```python
from build123d import *

# Parameters (mm, degrees)
F1_DEPTH = 9.8
F2_W     = 22.898962
F2_H     = 1.623713
F3_DEPTH = 18


with BuildPart() as f1:
    # F0 (on Top) → F1 (new body)
    with BuildSketch(Plane.XY):
        Polygon((30.061033, 31.619072), (-30.061033, 31.619072), (-16.680207, -13.655773), (-13.930722, -13.655773), (0, -13.655773), (13.930722, -13.655773), (16.680207, -13.655773), align=None)
        Polygon((-17.066102, 6.705488), (-22.912372, 26.4867), (22.912372, 26.4867), (17.066102, 6.705488), (0, 6.705488), align=None, mode=Mode.SUBTRACT)
        Polygon((0, -13.655773), (-13.930722, -13.655773), (-13.930722, -74.694335), (0, -74.694335), (13.930722, -74.694335), (13.930722, -13.655773), align=None)
    extrude(amount=F1_DEPTH)

    # F2 (on face) → F3 (cut)
    with BuildSketch(Plane(origin=(0, 6.705488, 0), x_dir=(-1, 0, 0), z_dir=(0, 1, 0))):
        with Locations((-0.274213, 4.465245)):
            Rectangle(F2_W, F2_H)
    extrude(amount=-F3_DEPTH, mode=Mode.SUBTRACT)


solid = f1.part
```
The model under review builds one solid part; all positions refer to its coordinate system, in mm. A direction names the side the tool comes from. Round coordinates to 2 decimals unless told otherwise and drop trailing zeros. Write each loop counter-clockwise with the first axis right and the second up, starting at its lowest first coordinate (ties: lowest second). Pieces come first, ordered by that corner, then holes. Notation, with made-up numbers: (-15.5, 9.25) - (-4.5, 9.25) arc R23 ccw to (-4.5, 45.25) - close; hole circle Ø11 at (78.25, -34.75). An arc over 180 degrees is marked (long way). One line per question, with ' | ' between items.
Item 1: Add section A-A, the plane x = 3.5. Give the boundary of the cut face in (y, z), then the cut area to 3 significant figures.
Resolved:
outline: (-74.69, 0) - (6.71, 0) - (6.71, 3.65) - (-11.29, 3.65) - (-11.29, 5.28) - (6.71, 5.28) - (6.71, 9.8) - (-74.69, 9.8) - close; (26.49, 0) - (31.62, 0) - (31.62, 9.8) - (26.49, 9.8) - close | area: 819 mm2
Item 2: Add section B-B, the plane y = 22. Give the boundary of the cut face in (x, z), then the cut area to 3 significant figures.
Resolved:
outline: (-27.22, 0) - (-21.59, 0) - (-21.59, 9.8) - (-27.22, 9.8) - close; (21.59, 0) - (27.22, 0) - (27.22, 9.8) - (21.59, 9.8) - close | area: 110 mm2
Item 3: For faces 1 (the face through (0, 26.487, 5)), 2 (the face through (13.931, -45, 5)), 3 (the face through (0, -74.694, 5)), 4 (the face through (0, -2, 5.277)), 5 (the face through (-13.931, -44, 5)), list the 3-axis set-ups (+Z, -Z, +X, -X, +Y, -Y) from which the entire face can be reached by the end or side of a thin tool; tool diameter is ignored.
Resolved:
face 1: +Z, -Z | face 2: +Z, -Z, +X, -Y | face 3: +Z, -Z, +X, -X, -Y | face 4: none | face 5: +Z, -Z, -X, -Y
Item 4: The part is to be moulded in two halves that separate along Y. For faces 6 (the face through (20.03, 16.73, 4.83)), 7 (the face through (-15, -13.656, 5)), 8 (the face through (0, -21, 9.8)), say which applies: pulls with the +Y half, pulls with the -Y half, needs draft (parallel to the pull), parting line crosses it, or undercut.
Resolved:
face 6: undercut | face 7: pulls with the -Y half | face 8: needs draft
Item 5: To check wall thickness, follow probe 1 along Y at (x, z) = (-10.5, 7.25); probe 2 along Y at (x, z) = (-16, 3.75); probe 3 along X at (y, z) = (-39.5, 7.25). State the ranges of each line that lie inside material, in increasing order.
Resolved:
probe 1: y = -74.69 to 6.71, 26.49 to 31.62 | probe 2: y = -13.66 to 6.71, 26.49 to 31.62 | probe 3: x = -13.93 to 13.93
Item 6: For P1, Ø3, axis at y = -29.5, z = 4.5, coming from the -X side; P2, Ø1.8, axis at y = 1.5, z = 4.5, coming from the -X side; P3, Ø5, axis at y = -48, z = 3.5, coming from the +X side, all flat-tipped, find the tip position at first contact; note any pin that passes through.
Resolved:
P1: stops at x = -13.93 | P2: stops at x = -21.43 | P3: stops at x = 13.93
Item 7: Add section C-C, the plane z = 1.75. Give the boundary of the cut face in (x, y), then the cut area to 3 significant figures.
Resolved:
outline: (-30.06, 31.62) - (-16.68, -13.66) - (-13.93, -13.66) - (-13.93, -74.69) - (13.93, -74.69) - (13.93, -13.66) - (16.68, -13.66) - (30.06, 31.62) - close; hole (-22.91, 26.49) - (-17.07, 6.71) - (17.07, 6.71) - (22.91, 26.49) - close | area: 3,030 mm2
Item 8: Add section D-D, the plane y = -56. Give the boundary of the cut face in (x, z), then the cut area to 3 significant figures.
Resolved:
outline: (-13.93, 0) - (13.93, 0) - (13.93, 9.8) - (-13.93, 9.8) - close | area: 273 mm2
